```python
from build123d import *

# Parameters (mm, degrees)
SKETCH1_R           = 10
SKETCH1_R_2         = 5.5
BOSS_EXTRUDE1_DEPTH = 3
BOSS_EXTRUDE2_START = -1
SKETCH2_R           = 12
SKETCH2_R_2         = 10
BOSS_EXTRUDE2_DEPTH = 1
SKETCH3_R           = 12
SKETCH3_R_2         = 10
BOSS_EXTRUDE3_DEPTH = 1
FILLET2_R           = 0.5


with BuildPart() as part:
    # Sketch1 → Boss-Extrude1 (new body)
    with BuildSketch(Plane(origin=(0, 0, 0), x_dir=(1, 0, 0), z_dir=(0, 1, 0))):
        with Locations(Location((0, 0, 0), (0, 0, 270))):
            Circle(SKETCH1_R)
        with Locations(Location((0, 0, 0), (0, 0, 270))):
            Circle(SKETCH1_R_2, mode=Mode.SUBTRACT)
    extrude(amount=BOSS_EXTRUDE1_DEPTH)

    # Sketch2 → Boss-Extrude2 (add)
    with BuildSketch(Plane(origin=(0, 3, 0), x_dir=(1, 0, 0), z_dir=(0, 1, 0)).offset(BOSS_EXTRUDE2_START)):
        with Locations(Location((0, 0, 0), (0, 0, 270))):
            Circle(SKETCH2_R)
        with Locations(Location((0, 0, 0), (0, 0, 270))):
            Circle(SKETCH2_R_2, mode=Mode.SUBTRACT)
    extrude(amount=BOSS_EXTRUDE2_DEPTH)

    # Sketch3 → Boss-Extrude3 (add)
    with BuildSketch(Plane.XZ):
        with Locations(Location((0, 0, 0), (0, 0, 90))):
            Circle(SKETCH3_R)
        with Locations(Location((0, 0, 0), (0, 0, 270))):
            Circle(SKETCH3_R_2, mode=Mode.SUBTRACT)
    extrude(amount=-BOSS_EXTRUDE3_DEPTH)

    # Fillet2
    fillet2_edges = [part.edges().sort_by_distance(p)[0] for p in [
        (0, 2, -10),
        (0, 1, -10),
    ]]
    fillet(fillet2_edges, radius=FILLET2_R - 0.0001)  # a hair under: the kernel refuses the full size


solid = part.part
```
Input: part model. Units: mm. Frame: model coordinates. A direction names the side the tool comes from. Round coordinates to 2 decimals unless told otherwise and drop trailing zeros. Loops run counter-clockwise (first coordinate to the right, second up) from the corner with the lowest first, then second, coordinate; pieces in that order, holes last. Notation, with made-up numbers: (-24.5, 83) -> (4.5, 83) arc R13 cw to (4.5, 88) -> close; hole circle Ø2 at (86.25, 0.25). An arc over 180 degrees is marked (long way). Use one line per item in the form item = value. Start each with the question number.
Item 1: Section query C-C on y = 2.45. Return the cut outline in (x, z).
Item 2: Set-up query: faces 4 (the face through (-11, 2, 0)), 5 (the face through (2.5, 0, 5.2)). Return all of +Z, -Z, +X, -X, +Y, -Y with unobstructed straight access to the full face (end or side cutting, diameter ignored); none if empty.
Item 3: Contact query for a flat-ended pin moving along its axis: pin 1 Ø9 at (x, z) = (0, 0) entering from +Y. Output: stop coordinate, or through.
Item 4: Material intervals for L1, parallel to Y at x = 11, z = 4; L2, parallel to X at y = 2.3, z = 0; L3, parallel to X at y = 1.45, z = 0, sorted ascending. Write a range as from..to.
Item 5: Mould query, pull axis Z, two halves, no side actions, for faces 1 (the face through (3.604, 2.493, 11.446)), 2 (the face through (11, 1, 0)), 3 (the face through (-5.37, 1.48, -1.19)). Classes: pulls with the +Z half, pulls with the -Z half, needs draft (parallel to the pull), parting line crosses it, or undercut.
Ans:
q1.outline = circle Ø24 at (0, 0); hole circle Ø11 at (0, 0)
q2.face_4 = none
q2.face_5 = +Z, -Z, +X, -X, -Y
q3.pin_1 = through
q4.L1 = 0..1, 2..3
q4.L2 = -12..-5.5, 5.5..12
q4.L3 = -10..-5.5, 5.5..10
q5.face_1 = parting line crosses it
q5.face_2 = needs draft
q5.face_3 = undercut
